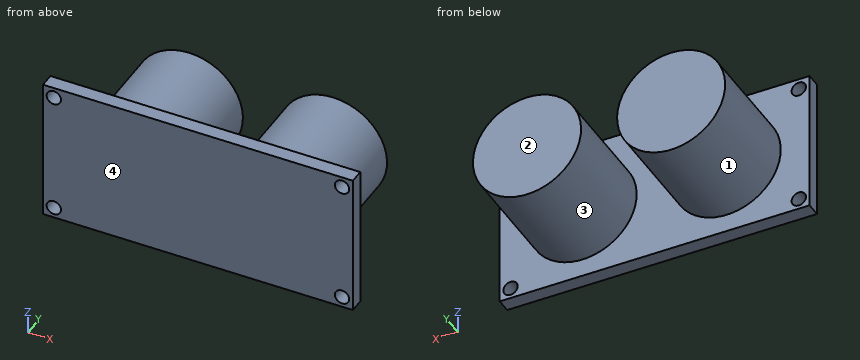
```python
from build123d import *

# Parameters (mm, degrees)
SKETCH1_W           = 43
SKETCH1_H           = 20
BOSS_EXTRUDE1_DEPTH = 2
SKETCH2_R           = 1
CUT_EXTRUDE1_DEPTH  = 2
SKETCH3_R           = 7.5
BOSS_EXTRUDE2_DEPTH = 15


with BuildPart() as part:
    # Sketch1 → Boss-Extrude1 (new body)
    with BuildSketch(Plane(origin=(0, 0, 0), x_dir=(1, 0, 0), z_dir=(0, 1, 0))):
        with Locations((1.884331799, -1.591272186)):
            Rectangle(SKETCH1_W, SKETCH1_H)
    extrude(amount=BOSS_EXTRUDE1_DEPTH)

    # Sketch2 → Cut-Extrude1 (cut)
    with BuildSketch(Plane(origin=(0, 2, 0), x_dir=(1, 0, 0), z_dir=(0, 1, 0))):
        with Locations(Location((-18.115668201, -10.091272186, 0), (0, 0, 270))):
            Circle(SKETCH2_R)
        with Locations(Location((21.884331799, -10.091272186, 0), (0, 0, 270))):
            Circle(SKETCH2_R)
        with Locations(Location((-18.115668201, 6.908727814, 0), (0, 0, 270))):
            Circle(SKETCH2_R)
        with Locations(Location((21.884331799, 6.908727814, 0), (0, 0, 270))):
            Circle(SKETCH2_R)
    extrude(amount=-CUT_EXTRUDE1_DEPTH, mode=Mode.SUBTRACT)

    # Sketch3 → Boss-Extrude2 (add)
    with BuildSketch(Plane(origin=(0, 2, 0), x_dir=(1, 0, 0), z_dir=(0, 1, 0))):
        with Locations(Location((11.884331799, -1.591272186, 0), (0, 0, 270))):
            Circle(SKETCH3_R)
        with Locations(Location((-8.115668201, -1.591272186, 0), (0, 0, 270))):
            Circle(SKETCH3_R)
    extrude(amount=BOSS_EXTRUDE2_DEPTH)


solid = part.part
```
Input: part model. Units: mm. Frame: model coordinates. Face numbers are marked on the shaded views. A direction names the side the tool comes from. Coordinates: 2 decimals unless noted, no trailing zeros. Order: outer loops, then holes, each group sorted by start corner. A loop starts at its lowest first (then second) coordinate and runs counter-clockwise, first axis right, second up. Notation, with made-up numbers: (-3.5, 37.5) - (19.5, 37.5) arc R31 ccw to (19.5, 76.5) - close; hole circle Ø10 at (-20, 40). An arc over 180 degrees is marked (long way). Put each result on its own line as item: value.
1. Cut plane B-B on y = 3.25. Return the cut outline in (x, z), then the cut area to 3 significant figures.
Report:
outline: circle Ø15 at (-8.12, 1.59); circle Ø15 at (11.88, 1.59)
area: 353 mm2
2. Cut plane C-C on x = 7.5. Return the cut outline in (y, z).
Report:
outline: (0, -8.41) - (2, -8.41) - (2, -4.49) - (17, -4.49) - (17, 7.68) - (2, 7.68) - (2, 11.59) - (0, 11.59) - close
3. Reachability of the marked faces 3 and 4 from +Z, -Z, +X, -X, +Y, -Y: full face, straight path, thin tool, end or side. Return the list, or none.
Report:
face 3: +Y
face 4: +Z, -Z, +X, -X, -Y
4. Contact query for flat-ended pins moving along their axis: pin 1 Ø1.2 at (x, z) = (21.88, 10.09) entering from +Y; pin 2 Ø1 at (x, y) = (-8, 7.5) entering from +Z; pin 3 Ø2.5 at (x, z) = (21.88, -6.91) entering from -Y; pin 4 Ø6 at (x, y) = (-2, 6.5) entering from +Z. Output: stop coordinate, or through.
Report:
pin 1: passes through
pin 2: stops at z = 9.09
pin 3: stops at y = 0
pin 4: stops at z = 8.41
5. Draft query along X for the marked faces 1 and 2. Return one class per face: pulls with the +X half, pulls with the -X half, needs draft (parallel to the pull), parting line crosses it, or undercut.
Report:
face 1: undercut
face 2: needs draft
6. Line query: line 1 along Y through (x, z) = (-17.5, -6); line 2 along X through (y, z) = (15.5, -3); line 3 along X through (y, z) = (4, 1.25). Output: solid intervals per line, ascending.
Report:
line 1: y = 0 to 2
line 2: x = -14.05 to -2.19, 5.95 to 17.81
line 3: x = -15.61 to -0.62, 4.39 to 19.38
7. Cut plane A-A on z = -3.75. Return the cut outline in (x, y), then the cut area to 3 significant figures.
Report:
outline: (-19.62, 0) - (23.38, 0) - (23.38, 2) - (17.15, 2) - (17.15, 17) - (6.62, 17) - (6.62, 2) - (-2.85, 2) - (-2.85, 17) - (-13.38, 17) - (-13.38, 2) - (-19.62, 2) - close
area: 402 mm2
8. Cut plane D-D on z = 0.75. Return the cut outline in (x, y), then the cut area to 3 significant figures.
Report:
outline: (-19.62, 0) - (23.38, 0) - (23.38, 2) - (19.34, 2) - (19.34, 17) - (4.43, 17) - (4.43, 2) - (-0.66, 2) - (-0.66, 17) - (-15.57, 17) - (-15.57, 2) - (-19.62, 2) - close
area: 533 mm2
